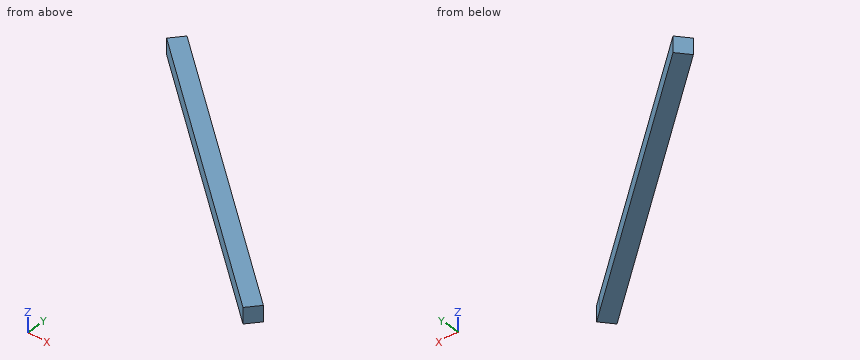
Autodesk Inventor part; units mm, degrees
ref_plane "Work Plane1" through (88.9, 0, 0) normal (1, 0, 0) x (0, 1, 0)
ref_plane "XZ Plane" through (0, 0, 0) normal (0, 1, 0) x (-1, 0, 0)
ref_plane "XY Plane" through (0, 0, 0) normal (0, 0, 1) x (1, 0, 0)
sketch "Sketch1" plane through (0, 0, 0) normal (0, 0, 1) x (1, 0, 0)
  line L0 (-351.8656, 461.0371) -> (76.2, 101.8473)
  line L1 (76.2, 135.0047) -> (-335.5388, 480.4946)
  line L2 (-335.5388, 480.4946) -> (-351.8656, 461.0371)
  line L3 (0, 0) -> (0, 391.6762) construction
  line L4 (76.2, 135.0047) -> (76.2, 101.8473)
  line L5 (76.2, 135.0047) -> (92.5268, 121.3049)
  line L6 (76.2, 101.8473) -> (92.5268, 121.3049)
  dimension "d29" = 76.2
  dimension "d30" = 558.8
extrude "Extrusion2" add sketch "Sketch1" along normal mid plane 25.4
ref_plane "Work Plane1" through (88.9, 0, 0) normal (1, 0, 0) x (0, 1, 0)
properties part number "newPullyV03"
Input: part model. Units: mm. Frame: model coordinates. Round coordinates to 2 decimals unless told otherwise and drop trailing zeros. Loops run counter-clockwise (first coordinate to the right, second up) from the corner with the lowest first, then second, coordinate; pieces in that order, holes last. Notation, with made-up numbers: (22.25, 25) -> (53.25, 25) arc R10 cw to (53.25, 38) -> close; hole circle Ø6 at (23, -16). An arc over 180 degrees is marked (long way). One line per item, written item: value.
(1) Material intervals for line 1 (X direction, y = 452, z = 4); line 2 (Y direction, x = -40.5, z = -7); line 3 (Y direction, x = -313, z = -9), sorted ascending. Write a range as [from, to].
Geometry check:
line 1: [-341.1, -301.58]
line 2: [199.77, 232.93]
line 3: [428.42, 461.58]
(2) Pin query (flat end, axial travel): pin 1 (10 mm diameter, centred on y = 423.5, z = -6.5, fed in from -X); pin 2 (2 mm diameter, centred on y = 145, z = 8.5, fed in from -X); pin 3 (2 mm diameter, centred on y = 354.5, z = -9.5, fed in from +X). Return the tip coordinate at first contact, or that it passes through.
Geometry check:
pin 1: x = -313.09
pin 2: x = 23.58
pin 3: x = -184.19
(3) Section A-A (z = -8.25). Return the cut outline in (x, y), plus the area to 3 significant figures.
Geometry check:
outline: (-351.87, 461.04) -> (76.2, 101.85) -> (92.53, 121.3) -> (76.2, 135) -> (-335.54, 480.49) -> close
area: 14,200 mm2
(4) Section C-C (x = -71). Return the cut outline in (y, z).
Geometry check:
outline: (225.36, -12.7) -> (258.52, -12.7) -> (258.52, 12.7) -> (225.36, 12.7) -> close
(5) Section B-B (y = 397.5). Return the cut outline in (x, z), plus the area to 3 significant figures.
Geometry check:
outline: (-276.15, -12.7) -> (-236.63, -12.7) -> (-236.63, 12.7) -> (-276.15, 12.7) -> close
area: 1,000 mm2
